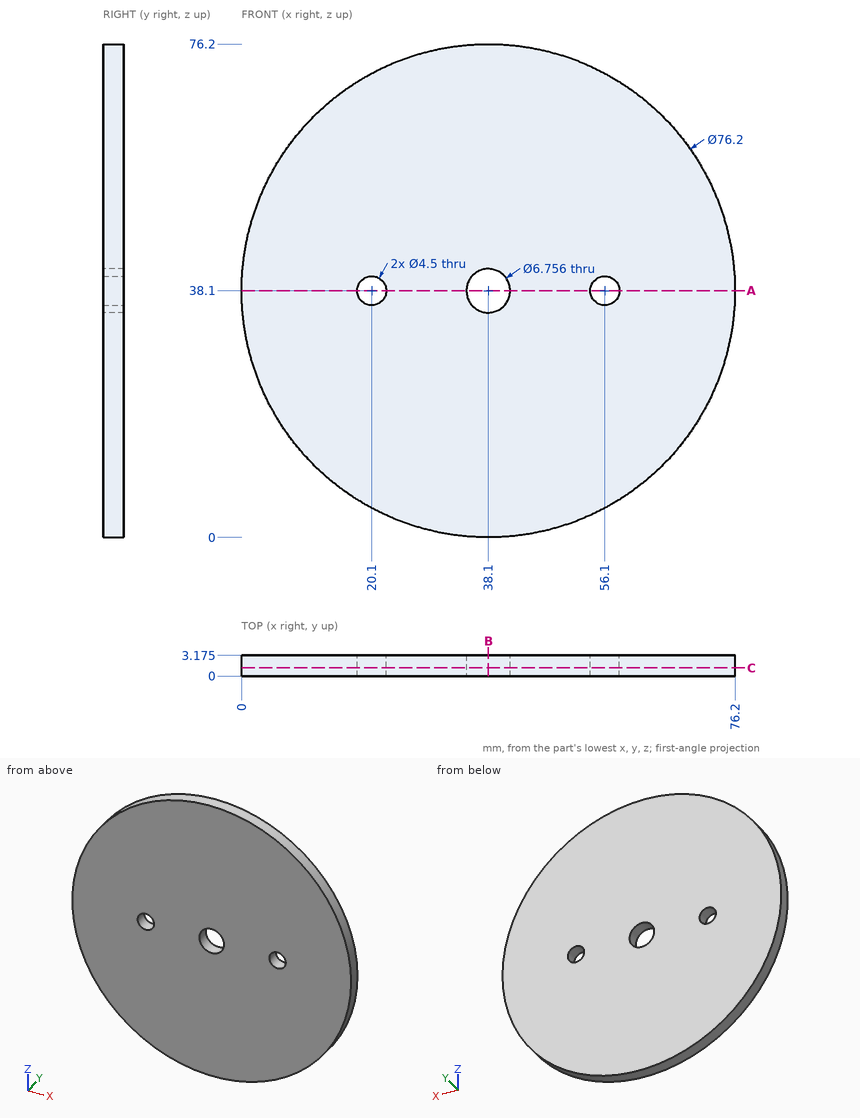
Study the drawing (mm; zero at the part's minimum x, y, z) and answer. Coordinates: 2 decimals unless noted, no trailing zeros. Order: outer loops, then holes, each group sorted by start corner. A loop starts at its lowest first (then second) coordinate and runs counter-clockwise, first axis right, second up. Notation, with made-up numbers: (75.5, 81) -> (108.5, 81) arc R7 ccw to (108.5, 88) -> close; hole circle Ø3 at (-12, 26.25). An arc over 180 degrees is marked (long way). Answer in a Markdown table with one row per item. Add a question column.
Item 1: Find section A-A (z = 38.1). State how many separate pieces and enclosed holes the cut face has, then the cut area to 3 significant figures.
Item 2: Find the intervals of material crossed by L1, parallel to X at y = 1.15, z = 37 (1 decimal); L2, parallel to Z at x = 38.1, y = 1; L3, parallel to Z at x = 20.1, y = 2.35, in increasing order. Write a range as from..to.
Item 3: Find section B-B (x = 38.1). Write down the section's boundary in (y, z) (1 decimal).
Item 4: Find section C-C (y = 1.25). Write down the section's boundary in (x, z).
Item 5: This flat-tipped pin is pushed along its axis until it touches: P1, Ø11, axis at x = 38.1, z = 38.1, coming from the +Y side (3 decimals). Where does it stop, or does it pass through?
Result set:
| question | item | result |
|---|---|---|
| 1 | separate pieces | 4 |
| 1 | enclosed holes | 0 |
| 1 | area | 192 mm² |
| 2 | L1 | x = 0..18.1, 22.1..34.9, 41.3..54.1, 58.1..76.2 |
| 2 | L2 | z = 0..34.72, 41.48..76.2 |
| 2 | L3 | z = 4.52..35.85, 40.35..71.68 |
| 3 | outline | (0, 0) -> (3.2, 0) -> (3.2, 34.7) -> (0, 34.7) -> close; (0, 41.5) -> (3.2, 41.5) -> (3.2, 76.2) -> (0, 76.2) -> close |
| 4 | outline | circle Ø76.2 at (38.1, 38.1); hole circle Ø4.5 at (20.1, 38.1); hole circle Ø6.76 at (38.1, 38.1); hole circle Ø4.5 at (56.1, 38.1) |
| 5 | P1 | stops at y = 3.175 |
